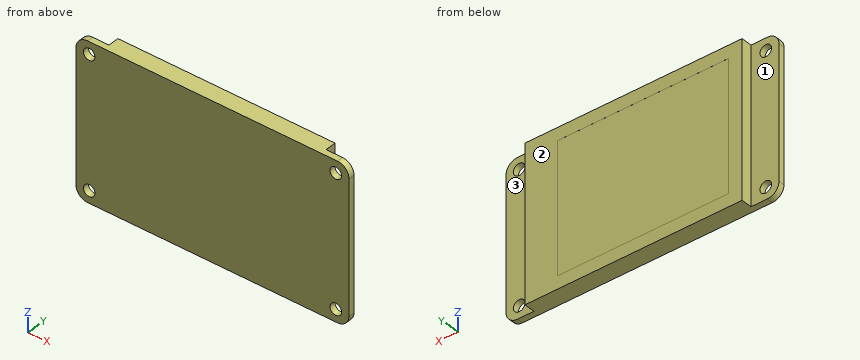
```python
from build123d import *

# Parameters (mm, degrees)
SKETCH_1_W          = 70.65
SKETCH_1_H          = 40.19
EXTRUDE_1_DEPTH     = 1.6
FILLET_1_R          = 3
SKETCH_2_R          = 1.5
CUT_EXTRUDE_1_DEPTH = 1.6
SKETCH_3_W          = 56.2
SKETCH_3_H          = 40.19
EXTRUDE_2_DEPTH     = 2.84
SKETCH_4_W          = 44.23
SKETCH_4_H          = 33.59
CUT_EXTRUDE_2_DEPTH = 0.01


with BuildPart() as part:
    # 草圖1 → 填料-伸長1 (new body)
    with BuildSketch(Plane(origin=(0, 0, 0), x_dir=(1, 0, 0), z_dir=(0, 1, 0))):
        with Locations((-2.656997534, 3.164617756)):
            Rectangle(SKETCH_1_W, SKETCH_1_H)
    extrude(amount=EXTRUDE_1_DEPTH)

    # 圓角1
    fillet_1_edges = [part.edges().sort_by_distance(p)[0] for p in [
        (-37.981997534, 0.8, -23.259617756),
        (32.668002466, 0.8, -23.259617756),
        (32.668002466, 0.8, 16.930382244),
        (-37.981997534, 0.8, 16.930382244),
    ]]
    fillet(fillet_1_edges, radius=FILLET_1_R)

    # 草圖2 → 除料-伸長1 (cut)
    with BuildSketch(Plane(origin=(0, 1.6, 0), x_dir=(1, 0, 0), z_dir=(0, 1, 0))):
        with Locations(Location((-34.561997534, 20.099617756, 0), (0, 0, 270))):
            Circle(SKETCH_2_R)
        with Locations(Location((29.248002466, 20.099617756, 0), (0, 0, 270))):
            Circle(SKETCH_2_R)
        with Locations(Location((-34.561997534, -13.770382244, 0), (0, 0, 270))):
            Circle(SKETCH_2_R)
        with Locations(Location((29.248002466, -13.770382244, 0), (0, 0, 270))):
            Circle(SKETCH_2_R)
    extrude(amount=-CUT_EXTRUDE_1_DEPTH, mode=Mode.SUBTRACT)

    # 草圖3 → 填料-伸長2 (add)
    with BuildSketch(Plane(origin=(0, 1.6, 0), x_dir=(1, 0, 0), z_dir=(0, 1, 0))):
        with Locations((-2.656997534, 3.164617756)):
            Rectangle(SKETCH_3_W, SKETCH_3_H)
    extrude(amount=EXTRUDE_2_DEPTH)

    # 草圖4 → 除料-伸長2 (cut)
    with BuildSketch(Plane(origin=(0, 4.44, 0), x_dir=(1, 0, 0), z_dir=(0, 1, 0))):
        with Locations((-5.081997534, 3.164617756)):
            Rectangle(SKETCH_4_W, SKETCH_4_H)
    extrude(amount=-CUT_EXTRUDE_2_DEPTH, mode=Mode.SUBTRACT)


solid = part.part
```
Model file for the job. Use its own axes, mm. Face numbers are marked on the shaded views. A direction names the side the tool comes from. Coordinates: 2 decimals unless noted, no trailing zeros. Write each loop counter-clockwise with the first axis right and the second up, starting at its lowest first coordinate (ties: lowest second). Pieces come first, ordered by that corner, then holes. Notation, with made-up numbers: (2, -6.75) - (6, -6.75) arc R14 ccw to (6, 13.25) - close; hole circle Ø11 at (42.5, -34.5). An arc over 180 degrees is marked (long way). Use a Markdown table: item, result. Add a question column.
Item 1: Drill centre lines: line 1 along Z through (x, y) = (-34, 1.2); line 2 along X through (y, z) = (2.45, -7); line 3 along Y through (x, z) = (28.5, 3.5). Where is each one in solid material? Low to high.
Item 2: 3-axis set-ups, long thin cutter, end or side, ignore diameter. For the marked faces 1, 2 and 3: which of +Z, -Z, +X, -X, +Y, -Y reach the whole face in a straight line?
Item 3: Drop flat-ended pins along their axis: pin 1 (1 mm diameter, centred on y = 3, z = -19, fed in from -X); pin 2 (4 mm diameter, centred on x = -34.56, z = 13.77, fed in from +Y); pin 3 (2.5 mm diameter, centred on x = 29.25, z = -20.1, fed in from -Y); pin 4 (5 mm diameter, centred on x = -23.5, z = 6, fed in from +Y). Give the stop position or say it passes through.
Item 4: Band-saw the part on B-B, the plane y = 2.45. Write the cut outline in (x, z), and give its area (3 significant figures).
A:
| question | item | result |
|---|---|---|
| 1 | line 1 | z = -23.26 to -21.49, -18.71 to 12.38, 15.16 to 16.93 |
| 1 | line 2 | x = -30.76 to 25.44 |
| 1 | line 3 | y = 0 to 1.6 |
| 2 | face 1 | +Z, -Z, -X, +Y |
| 2 | face 2 | +Z, -Z, +X, -X, +Y |
| 2 | face 3 | +Z, -Z, +X, +Y |
| 3 | pin 1 | stops at x = -30.76 |
| 3 | pin 2 | stops at y = 1.6 |
| 3 | pin 3 | passes through |
| 3 | pin 4 | stops at y = 4.43 |
| 4 | outline | (-30.76, -23.26) - (25.44, -23.26) - (25.44, 16.93) - (-30.76, 16.93) - close |
| 4 | area | 2,260 mm² |
